Geometry check sheet. Reference: the model listing, model coordinates, mm. Coordinates: 2 decimals unless noted, no trailing zeros. Loops run counter-clockwise (first coordinate to the right, second up) from the corner with the lowest first, then second, coordinate; pieces in that order, holes last. Notation, with made-up numbers: (-28.5, 38) - (20.5, 38) arc R23 ccw to (20.5, 54) - close; hole circle Ø5 at (31, 58.5). An arc over 180 degrees is marked (long way). Write each question's results on one line, items separated by ' | '. Start each with the question number.
(1) Sectioned sample at B-B (z = -42). Enter the section's corners in (x, y).
(2) Sectioned sample at A-A (x = 276). Enter the section's corners in (y, z).
(3) Material ranges on probe 1 along Y at (x, z) = (158, -29.5); probe 2 along Y at (x, z) = (224, -7); probe 3 along X at (y, z) = (10, -35.5), recorded low to high.
(4) Go/stop test with flat-tipped pins: pin 1 Ø1.6 at (y, z) = (8.5, -27.5) entering from -X; pin 2 Ø5 at (x, z) = (268, -17.5) entering from +Y; pin 3 Ø2 at (y, z) = (8.5, -20.5) entering from -X. Record where each tip stops, or that it passes through.
from build123d import *

# Parameters (mm, degrees)
BOSS_EXTRUDE1_DEPTH = 300
SKETCH2_R           = 1
SKETCH2_W           = 2
SKETCH2_H           = 2
BOSS_EXTRUDE2_DEPTH = 2.5
FILLET1_R           = 5
FILLET2_R           = 0.5


# Read off the part's stored shape, not the designer's step: Boss-Extrude1
with BuildPart() as part:
    # Boss-Extrude1 outline → Boss-Extrude1 (new body)
    with BuildSketch(Plane.YZ):
        Polygon((0, -70), (11.580431243, -70), (4.223134774, 0), (0, 0), align=None)
    extrude(amount=BOSS_EXTRUDE1_DEPTH)

    # Sketch2 → Boss-Extrude2 (add)
    with BuildSketch(Plane(origin=(0, 4.176991961, 0.439019546), x_dir=(-1, 0, 0), z_dir=(0, 0.9945218953682733, 0.10452846326765368))):
        with Locations((-140.1, -22.641437788)):
            Circle(SKETCH2_R)
        with BuildLine():
            ThreePointArc((-141.1, -22.641437788), (-140.1, -21.641437788), (-139.1, -22.641437788))
            Line((-139.1, -22.641437788), (-139.1, -20.141437788))
            ThreePointArc((-139.1, -20.141437788), (-140.1, -21.141437788), (-141.1, -20.141437788))
            Line((-141.1, -20.141437788), (-141.1, -22.641437788))
        make_face()
        with Locations((-140.1, -20.141437788)):
            Circle(SKETCH2_R)
        with Locations((-143.6, -20.141437788)):
            Circle(SKETCH2_R)
        with BuildLine():
            ThreePointArc((-144.6, -30.641437788), (-143.6, -29.641437788), (-142.6, -30.641437788))
            Line((-142.6, -30.641437788), (-142.6, -20.141437788))
            ThreePointArc((-142.6, -20.141437788), (-143.6, -21.141437788), (-144.6, -20.141437788))
            Line((-144.6, -20.141437788), (-144.6, -30.641437788))
        make_face()
        with Locations((-143.6, -30.641437788)):
            Circle(SKETCH2_R)
        with Locations(Location((-143.6, -34.141437788, 0), (0, 0, 90))):
            Circle(SKETCH2_R)
        with Locations((-148.1, -38.141437788)):
            Circle(SKETCH2_R)
        with BuildLine():
            ThreePointArc((-149.1, -38.141437788), (-148.1, -37.141437788), (-147.1, -38.141437788))
            Line((-147.1, -38.141437788), (-147.1, -35.141437788))
            Line((-147.1, -35.141437788), (-149.1, -35.141437788))
            Line((-149.1, -35.141437788), (-149.1, -38.141437788))
        make_face()
        with Locations((-148.1, -34.141437788)):
            Rectangle(SKETCH2_W, SKETCH2_H)
        with BuildLine():
            Line((-149.1, -33.141437788), (-147.1, -33.141437788))
            Line((-147.1, -33.141437788), (-147.1, -24.141437788))
            ThreePointArc((-147.1, -24.141437788), (-148.1, -25.141437788), (-149.1, -24.141437788))
            Line((-149.1, -24.141437788), (-149.1, -33.141437788))
        make_face()
        with Locations((-148.1, -24.141437788)):
            Circle(SKETCH2_R)
        with Locations((-151.1, -34.141437788)):
            Circle(SKETCH2_R)
        with BuildLine():
            Line((-151.1, -35.141437788), (-149.1, -35.141437788))
            Line((-149.1, -35.141437788), (-149.1, -33.141437788))
            Line((-149.1, -33.141437788), (-151.1, -33.141437788))
            ThreePointArc((-151.1, -33.141437788), (-150.392893219, -33.434331007), (-150.1, -34.141437788))
            ThreePointArc((-150.1, -34.141437788), (-150.392893219, -34.848544569), (-151.1, -35.141437788))
        make_face()
        with Locations((-152.9, -30.641437788)):
            Circle(SKETCH2_R)
        with BuildLine():
            ThreePointArc((-153.9, -30.641437788), (-152.9, -29.641437788), (-151.9, -30.641437788))
            Line((-151.9, -30.641437788), (-151.9, -24.641437788))
            ThreePointArc((-151.9, -24.641437788), (-152.9, -25.641437788), (-153.9, -24.641437788))
            Line((-153.9, -24.641437788), (-153.9, -30.641437788))
        make_face()
        with Locations((-152.9, -24.641437788)):
            Circle(SKETCH2_R)
        with Locations((-156.4, -30.641437788)):
            Circle(SKETCH2_R)
        with Locations((-156.4, -24.641437788)):
            Circle(SKETCH2_R)
        with Locations((-159.9, -30.641437788)):
            Circle(SKETCH2_R)
        with Locations((-159.9, -24.641437788)):
            Circle(SKETCH2_R)
        with BuildLine():
            ThreePointArc((-157.4, -30.641437788), (-156.4, -29.641437788), (-155.4, -30.641437788))
            Line((-155.4, -30.641437788), (-155.4, -24.641437788))
            ThreePointArc((-155.4, -24.641437788), (-156.4, -25.641437788), (-157.4, -24.641437788))
            Line((-157.4, -24.641437788), (-157.4, -30.641437788))
        make_face()
        with BuildLine():
            ThreePointArc((-160.9, -30.641437788), (-159.9, -29.641437788), (-158.9, -30.641437788))
            Line((-158.9, -30.641437788), (-158.9, -24.641437788))
            ThreePointArc((-158.9, -24.641437788), (-159.9, -25.641437788), (-160.9, -24.641437788))
            Line((-160.9, -24.641437788), (-160.9, -30.641437788))
        make_face()
    extrude(amount=BOSS_EXTRUDE2_DEPTH)

    # Fillet1
    fillet1_edges = [part.edges().sort_by_distance(p)[0] for p in [
        (300, 5.790215621, -70),
        (300, 2.111567387, 0),
        (0, 2.111567387, 0),
        (0, 5.790215621, -70),
    ]]
    fillet(fillet1_edges, radius=FILLET1_R)

    # Fillet2
    fillet2_edges = [part.edges().sort_by_distance(p)[0] for p in [
        (149.1, 8.884367892, -32.390205399),
        (149.1, 9.093424819, -34.37924919),
    ]]
    fillet(fillet2_edges, radius=FILLET2_R)


solid = part.part
Outcome:
1) outline: (0, 0) - (300, 0) - (300, 8.64) - (0, 8.64) - close
2) outline: (0, -70) - (11.58, -70) - (4.22, 0) - (0, 0) - close
3) probe 1: y = 0 to 7.32 | probe 2: y = 0 to 4.96 | probe 3: x = 147.1 to 149.1
4) pin 1: stops at x = 142.6 | pin 2: stops at y = 6.33 | pin 3: stops at x = 139.1
